For this review, use the dimensioned drawing (mm, ordinates from the lowest corner) and the shaded views. Give positions to 0.01 mm unless a question says otherwise; leave off trailing zeros. Loops run counter-clockwise (first coordinate to the right, second up) from the corner with the lowest first, then second, coordinate; pieces in that order, holes last. Notation, with made-up numbers: M -32.75,86.25 L 4.25,86.25 A14 ccw 4.25,110.25 Z; hole C 28.25,-22 d10. An arc over 180 degrees is marked long. Return JSON: item names as keys, results as strings.
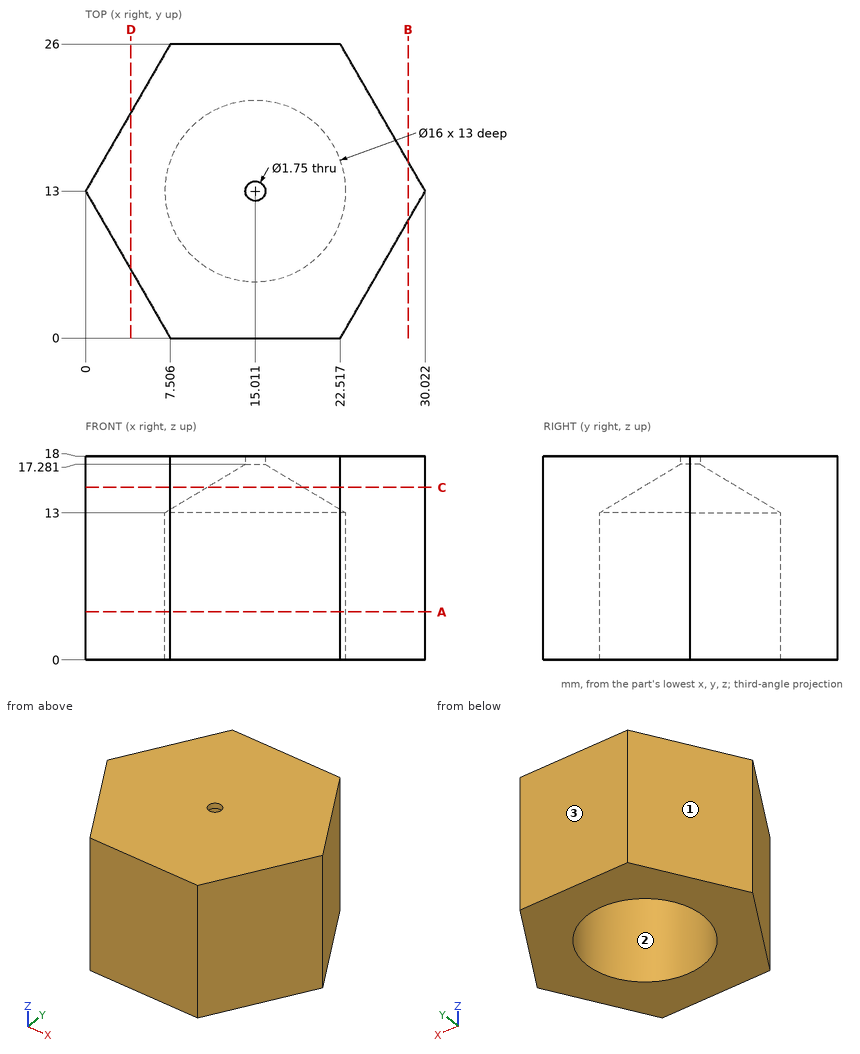
1) Consider section A-A on z = 4.25. Write out the cut boundary in (x, y) (1 decimal), then the cut area to 3 significant figures.
From the geometry:
{"outline": "M 0,13 L 7.5,0 L 22.5,0 L 30,13 L 22.5,26 L 7.5,26 Z; hole C 15,13 d16", "area": "384 mm²"}
2) Consider section B-B on x = 28.5. Write out the cut boundary in (y, z).
From the geometry:
{"outline": "M 10.36,0 L 15.64,0 L 15.64,18 L 10.36,18 Z"}
3) Consider section C-C on z = 15.25. Write out the cut boundary in (x, y) (1 decimal).
From the geometry:
{"outline": "M 0,13 L 7.5,0 L 22.5,0 L 30,13 L 22.5,26 L 7.5,26 Z; hole C 15,13 d8.5"}
4) Insertion check: pin 1 (5 mm diameter, centred on y = 20.5, z = 7, fed in from -X); pin 2 (10 mm diameter, centred on x = 6.5, z = 15.5, fed in from +Y); pin 3 (2.5 mm diameter, centred on x = 15.01, y = 13, fed in from -Z) (1 decimal); pin 4 (1.5 mm diameter, centred on y = 3, z = 5.5, fed in from -X). Each pin has a flat end and moves straight along its axis. Give the tip position at first contact, or say it passes through.
From the geometry:
{"pin 1": "x = 2.89", "pin 2": "y = 26", "pin 3": "z = 17.1", "pin 4": "x = 5.34"}
5) Consider section D-D on x = 4. Write out the cut boundary in (y, z), then the cut area to 3 significant figures.
From the geometry:
{"outline": "M 6.07,0 L 19.93,0 L 19.93,18 L 6.07,18 Z", "area": "249 mm²"}
6) Wall thickness on L1, parallel to X at y = 13, z = 17.7 (1 decimal); L2, parallel to X at y = 13, z = 10; L3, parallel to Y at x = 17, z = 2.5: over which ranges is each line inside the solid? List them lowest first. Write a range as from..to.
From the geometry:
{"L1": "0..14.1, 15.9..30", "L2": "0..7.01, 23.01..30.02", "L3": "0..5.25, 20.75..26"}
7) The part is to be moulded in two halves that separate along X. For the marked faces 1, 2 and 3, say which applies: released by +X, released by -X, zero draft, split by the parting line, or undercut.
From the geometry:
{"face 1": "released by -X", "face 2": "undercut", "face 3": "zero draft"}
